```python
from build123d import *

# Parameters (mm, degrees)
SKETCH004_W             = 51
SKETCH004_H             = 21
SKETCH004_R             = 1
PAD003_DEPTH            = 1
SKETCH005_W             = 6
SKETCH005_H             = 8
SKETCH005_W_2           = 4
SKETCH005_H_2           = 3
PAD004_DEPTH            = 3
SKETCH006_W             = 7
SKETCH006_H             = 7
PAD005_DEPTH            = 1
BODY001_PLACEMENT_ANGLE = 180


with BuildPart() as part:
    # Sketch004 → Pad003 (new body)
    with BuildSketch(Plane.XY):
        with Locations((-25.5, 10.5)):
            Rectangle(SKETCH004_W, SKETCH004_H)
        with Locations((-49, 16.2)):
            Circle(SKETCH004_R, mode=Mode.SUBTRACT)
        with Locations((-49, 4.8)):
            Circle(SKETCH004_R, mode=Mode.SUBTRACT)
        with Locations((-2, 16.2)):
            Circle(SKETCH004_R, mode=Mode.SUBTRACT)
        with Locations((-2, 4.8)):
            Circle(SKETCH004_R, mode=Mode.SUBTRACT)
    extrude(amount=PAD003_DEPTH)

    # Sketch005 (on Face10 of Pad003) → Pad004 (join)
    with BuildSketch(Plane.XY.offset(1)):
        with Locations((-1, 10.5)):
            Rectangle(SKETCH005_W, SKETCH005_H)
        with Locations((-11.248037, 13.892912)):
            Rectangle(SKETCH005_W_2, SKETCH005_H_2)
    extrude(amount=PAD004_DEPTH)

    # Sketch006 (on Face5 of Pad004) → Pad005 (join)
    with BuildSketch(Plane.XY.offset(1)):
        with Locations((-28.391885, 12.32462)):
            Rectangle(SKETCH006_W, SKETCH006_H)
    extrude(amount=PAD005_DEPTH)


with BuildPart() as part_1:
    # Body001 placement: moved
    add(part.part.moved(Location((-2, 46.5, -8))).rotate(Axis((-2, 46.5, -8), (0, 0, 1)), BODY001_PLACEMENT_ANGLE))


solid = part_1.part
```
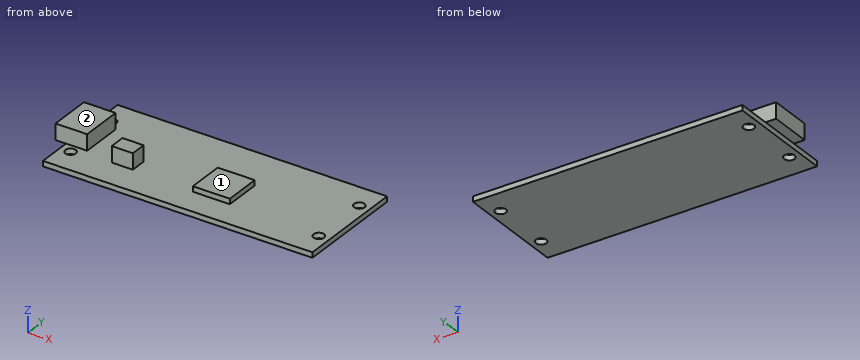
Geometry: final body of the model. Coordinates: model frame, mm. Face numbers are marked on the shaded views. A direction names the side the tool comes from. Coordinates: 2 decimals unless noted, no trailing zeros. Order: outer loops, then holes, each group sorted by start corner. A loop starts at its lowest first (then second) coordinate and runs counter-clockwise, first axis right, second up. Notation, with made-up numbers: M 60,3.5 L 80,3.5 A27 cw 80,24.5 Z; hole C 88.5,51.25 d3. An arc over 180 degrees is marked long. Answer as CSV lines item,"result".
Q1. Section B-B on z = -5.4. Return the cut outline in (x, y), and give its area (3 significant figures).
Answers:
outline,"M -4,32 L 2,32 L 2,40 L -4,40 Z; M 7.25,31.11 L 11.25,31.11 L 11.25,34.11 L 7.25,34.11 Z"
area,"60.0 mm^2"
Q2. Section A-A on x = 0. Return the cut outline in (y, z), and give its area (3 significant figures).
Answers:
outline,"M 25.5,-8 L 29.3,-8 L 29.3,-7 L 25.5,-7 Z; M 31.3,-8 L 40.7,-8 L 40.7,-7 L 40,-7 L 40,-4 L 32,-4 L 32,-7 L 31.3,-7 Z; M 42.7,-8 L 46.5,-8 L 46.5,-7 L 42.7,-7 Z"
area,"41.0 mm^2"
Q3. Line query: probe 1 along Y at (x, z) = (47, -7.5); probe 2 along X at (y, z) = (41.7, -7.2); probe 3 along X at (y, z) = (36.75, -7.7). Output: solid intervals per line, ascending. Write a range as [from, to].
Answers:
probe 1,"y = [25.5, 29.3], [31.3, 40.7], [42.7, 46.5]"
probe 2,"x = [-2, -1], [1, 46], [48, 49]"
probe 3,"x = [-2, 49]"
Q4. Set-up query: the marked faces 1 and 2. Return all of +Z, -Z, +X, -X, +Y, -Y with unobstructed straight access to the full face (end or side cutting, diameter ignored); none if empty.
Answers:
face 1,"+Z, +X, +Y, -Y"
face 2,"+Z, +X, -X, +Y, -Y"
Q5. Section D-D on x = 47. Return the cut outline in (y, z), and give its area (3 significant figures).
Answers:
outline,"M 25.5,-8 L 29.3,-8 L 29.3,-7 L 25.5,-7 Z; M 31.3,-8 L 40.7,-8 L 40.7,-7 L 31.3,-7 Z; M 42.7,-8 L 46.5,-8 L 46.5,-7 L 42.7,-7 Z"
area,"17.0 mm^2"
Q6. Section C-C on x = 9. Return the cut outline in (y, z), and give its area (3 significant figures).
Answers:
outline,"M 25.5,-8 L 46.5,-8 L 46.5,-7 L 34.11,-7 L 34.11,-4 L 31.11,-4 L 31.11,-7 L 25.5,-7 Z"
area,"30.0 mm^2"
Q7. First-contact query: P1, Ø1, axis at x = 36, y = 38.5, coming from the +Z side; P2, Ø1.8, axis at x = 47, y = 30.3, coming from the -Z side; P3, Ø1.1, axis at x = 25.5, z = -6.5, coming from the +Y side; P4, Ø1, axis at x = -3, y = 34, coming from the -Z side. Flat tips, straight axial feed; report the tip coordinate or a pass-through.
Answers:
P1,"stops at z = -7"
P2,"passes through"
P3,"stops at y = 46.5"
P4,"stops at z = -7"
